Could you check a few things on this model? Use its own coordinates, in mm. A direction names the side the tool comes from. Round coordinates to 2 decimals unless told otherwise and drop trailing zeros. Write each loop counter-clockwise with the first axis right and the second up, starting at its lowest first coordinate (ties: lowest second). Pieces come first, ordered by that corner, then holes. Notation, with made-up numbers: (-2, 84.5) -> (31, 84.5) arc R13 cw to (31, 104.5) -> close; hole circle Ø8 at (3, 5.25). An arc over 180 degrees is marked (long way). Answer as CSV lines item,"result". Start each with the question number.
Q1. Will these pins go through, and if not, where does the flat tip stop? pin 1 Ø10 at (x, z) = (65, 584) entering from -Y; pin 2 Ø1.9 at (x, z) = (2, 1097) entering from +Y; pin 3 Ø1.1 at (x, y) = (55.5, -1) entering from -Z; pin 4 Ø1.9 at (y, z) = (-1.5, 1107) entering from -X.
Q2. Imagine slicing it at B-B on x = 27.5. Please give me the cut outline in (y, z).
Q3. For faces 1 (the flat face through (41, -3.81, 551)), 2 (the flat face through (0, -41, 551)), which set-ups out of +Z, -Z, +X, -X, +Y, -Y let a thin tool reach every point of the face, with its end or its side?
Q4. Imagine slicing it at C-C on y = -51. Please give me the cut outline in (x, z).
Q5. If I drill on line 1 (X direction, y = -17, z = 1032); line 2 (Y direction, x = 64.5, z = 1008); line 3 (Y direction, x = 3.5, z = 430), over which ranges is the centre line in solid material (lowest first)? Write a range as [from, to].
from build123d import *

# Parameters (mm, degrees)
F1_DEPTH  = 1117.6
F1_FACE_W = 69.215
F1_FACE_H = 1117.6
F2_DEPTH  = 12.7
F3_W      = 4.401298
F3_H      = 9.729863
F3_W_2    = 12.7
F3_H_2    = 12.7
F4_DEPTH  = 3.811
F5_W      = 12.7
F5_H      = 12.7
F6_DEPTH  = 3.811
F7_W      = 12.7
F7_H      = 12.7
F8_DEPTH  = 3.811


with BuildPart() as f1:
    # F0 (on Top) → F1 (new body)
    with BuildSketch(Plane.XY):
        with BuildLine():
            ThreePointArc((0, -75.3745), (0.241783, -75.958217), (0.8255, -76.2))
            Line((0.8255, -76.2), (3.81, -76.2))
            Line((3.81, -76.2), (3.81, -6.985))
            ThreePointArc((3.81, -6.985), (4.739936, -4.739936), (6.985, -3.81))
            Line((6.985, -3.81), (76.2, -3.81))
            Line((76.2, -3.81), (76.2, -0.8255))
            ThreePointArc((76.2, -0.8255), (75.958217, -0.241783), (75.3745, 0))
            Line((75.3745, 0), (6.985, 0))
            ThreePointArc((6.985, 0), (2.045859, -2.045859), (0, -6.985))
            Line((0, -6.985), (0, -75.3745))
        make_face()
    extrude(amount=F1_DEPTH)

    # F1_face (on face) → F2 (cut)
    with BuildSketch(Plane(origin=(41.5925, -3.81, 558.8), x_dir=(1, 0, 0), z_dir=(0, -1, 0))):
        Rectangle(F1_FACE_W, F1_FACE_H)
    extrude(amount=F2_DEPTH, mode=Mode.SUBTRACT)

    # F3 (on face) → F4 (cut, through all)
    with BuildSketch(Plane.XZ.offset(3.81)):
        with Locations((15.575112, 1109.140038)):
            Rectangle(F3_W, F3_H)
        with Locations((45.943957, 1106.071313)):
            Rectangle(F3_W_2, F3_H_2)
    extrude(amount=-F4_DEPTH, mode=Mode.SUBTRACT)

    # F5 (on face) → F6 (cut, through all)
    with BuildSketch(Plane.YZ.offset(3.81)):
        with Locations((-29.260806, 1094.573338)):
            Rectangle(F5_W, F5_H)
    extrude(amount=-F6_DEPTH, mode=Mode.SUBTRACT)

    # F7 (on face) → F8 (cut, through all)
    with BuildSketch(Plane.XZ.offset(3.81)):
        with Locations((55.762946, 17.327846)):
            Rectangle(F7_W, F7_H)
    extrude(amount=-F8_DEPTH, mode=Mode.SUBTRACT)


solid = f1.part
Checks:
1,pin 1,"y = -3.81"
1,pin 2,"y = -1.28"
1,pin 3,"z = 0"
1,pin 4,"x = 1.67"
2,outline,"(-3.81, 0) -> (0, 0) -> (0, 1117.6) -> (-3.81, 1117.6) -> close"
3,face 1,"+Z, -Z, +X, -Y"
3,face 2,"+Z, -Z, -X, +Y, -Y"
4,outline,"(0, 0) -> (3.81, 0) -> (3.81, 1117.6) -> (0, 1117.6) -> close"
5,line 1,"[0, 3.81]"
5,line 2,"[-3.81, 0]"
5,line 3,"[-76.2, -0.93]"
